Geometry: final body of the model. Coordinates: model frame, mm. Face numbers are marked on the shaded views. A direction names the side the tool comes from. Give positions to 0.01 mm unless a question says otherwise; leave off trailing zeros. Loops run counter-clockwise (first coordinate to the right, second up) from the corner with the lowest first, then second, coordinate; pieces in that order, holes last.
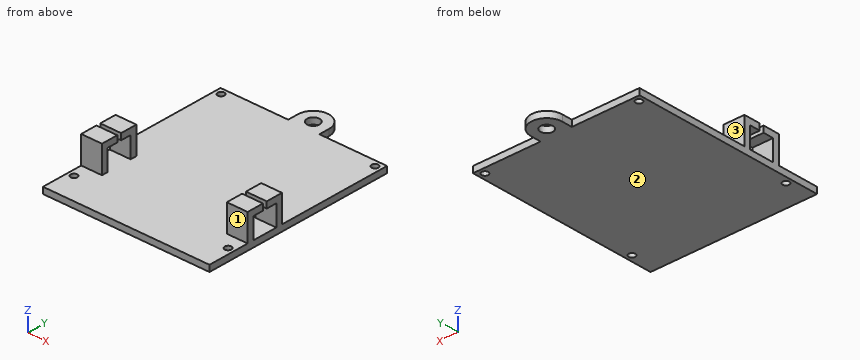
Autodesk Inventor part; units mm, degrees
ref_plane "YZ Plane" through (0, 0, 0) normal (1, 0, 0) x (0, 1, 0)
ref_plane "XZ Plane" through (0, 0, 0) normal (0, 1, 0) x (-1, 0, 0)
ref_plane "XY Plane" through (0, 0, 0) normal (0, 0, 1) x (1, 0, 0)
sketch "Sketch1" plane through (0, 0, 0) normal (0, 0, 1) x (1, 0, 0)
  line L0 (0, 0) -> (80, 0)
  line L1 (80, 0) -> (80, 93)
  line L2 (80, 93) -> (0, 93)
  line L3 (0, 93) -> (0, 0)
  dimension "d0" = 80
  dimension "d1" = 93
extrude "Extrusion1" add sketch "Sketch1" along normal blind 3
sketch "Sketch3" plane through (80, 0, 0) normal (1, 0, 0) x (0, 0, -1)
  line L0 (-3, 0) -> (-3, 93) construction
  line L1 (-3, 20) -> (-16, 20)
  line L2 (-16, 38) -> (-3, 38)
  line L3 (-3, 38) -> (-3, 20) construction
  line L4 (-3, 23) -> (-13, 23)
  line L5 (-13, 35) -> (-3, 35)
  line L6 (0, 0) -> (-3, 0)
  line L7 (-16, 28) -> (-13, 28)
  line L8 (-13, 30) -> (-16, 30)
  line L9 (-16, 20) -> (-16, 28)
  line L10 (-16, 30) -> (-16, 38)
  line L11 (-13, 23) -> (-13, 28)
  line L12 (-13, 30) -> (-13, 35)
  line L13 (-3, 38) -> (-3, 35)
  line L14 (-3, 20) -> (-3, 23)
  point P0 (-13, 19)
  point P1 (-16, 19)
  dimension "d4" = 3
  dimension "d6" = 20
  dimension "d7" = 12
  dimension "d8" = 10
  dimension "d9" = 3
  dimension "d10" = 5
  dimension "d11" = 5
  dimension "d12" = 3
ref_plane "Work Plane1" through (40, 0, 0) normal (1, 0, 0) x (0, 0, -1)
extrude "Extrusion2" add sketch "Sketch3" against normal blind 10
mirror "Mirror1" about plane through (40, 0, 0) normal (1, 0, 0) of "Extrusion2"
sketch "Sketch4" plane through (0, 0, 3) normal (0, 0, 1) x (1, 0, 0)
  circle A0 centre (77, 13) radius 1.6
  line L0 (80, 0) -> (80, 20)
  line L1 (0, 0) -> (80, 0)
  circle A1 centre (77, 90) radius 1.6
  line L2 (80, 93) -> (0, 93)
  dimension "d15" = 3.2
  dimension "d16" = 3
  dimension "d17" = 13
  dimension "d18" = 3
extrude "Extrusion3" cut sketch "Sketch4" against normal through all
mirror "Mirror2" about plane through (40, 0, 0) normal (1, 0, 0) of "Extrusion2", "Extrusion3"
sketch "Sketch5" plane through (0, 0, 0) normal (0, 0, -1) x (-1, 0, 0)
  line L0 (-80, 93) -> (0, 93) construction
  line L1 (-47.5, 93) -> (-32.5, 93)
  line L2 (-32.5, 93) -> (-32.5, 98)
  line L3 (-32.5, 98) -> (-47.5, 98) construction
  line L4 (-47.5, 98) -> (-47.5, 93)
  arc A0 (-32.5, 98) -> (-47.5, 98) centre (-40, 98) ccw
  circle A1 centre (-40, 98) radius 3
  point P0 (0, 0)
  point P1 (-40, 93)
  point P2 (-40, 93)
  dimension "d21" = 6
  dimension "d22" = 15
  dimension "d23" = 5
extrude "Extrusion4" add sketch "Sketch5" against normal blind 3
equation "\"d11\" = d10"
equation "\"d12\" = d4"
equation "\"d18\" = d16"
equation "\"d5\" = d4"
properties part number "Wheel Base"
Item 1: Ray query, probe 1 along Y at (x, z) = (77, 2.35); probe 2 along X at (y, z) = (90, 1.2); probe 3 along Y at (x, z) = (6.5, 4.25). Return the intervals inside material, ascending.
Values follow:
probe 1: y = 0 to 11.4, 14.6 to 88.4, 91.6 to 93
probe 2: x = 0 to 1.4, 4.6 to 75.4, 78.6 to 80
probe 3: y = 20 to 23, 35 to 38
Item 2: Section query D-D on x = 40. Return loops of the section in (y, z).
Values follow:
outline: (0, 0) - (95, 0) - (95, 3) - (0, 3) - close; (101, 0) - (105.5, 0) - (105.5, 3) - (101, 3) - close
Item 3: Set-up query: the marked faces 1, 2 and 3. Return all of +Z, -Z, +X, -X, +Y, -Y with unobstructed straight access to the full face (end or side cutting, diameter ignored); none if empty.
Values follow:
face 1: +Z, +X, -X, -Y
face 2: -Z, +X, -X, +Y, -Y
face 3: +Z, +X, -X, +Y
Item 4: Section query A-A on y = 90. Return loops of the section in (x, z), plus the area to 3 significant figures.
Values follow:
outline: (0, 0) - (1.4, 0) - (1.4, 3) - (0, 3) - close; (4.6, 0) - (75.4, 0) - (75.4, 3) - (4.6, 3) - close; (78.6, 0) - (80, 0) - (80, 3) - (78.6, 3) - close
area: 221 mm2
Item 5: Section query C-C on x = 77. Return loops of the section in (y, z).
Values follow:
outline: (0, 0) - (11.4, 0) - (11.4, 3) - (0, 3) - close; (14.6, 0) - (88.4, 0) - (88.4, 3) - (38, 3) - (38, 16) - (30, 16) - (30, 13) - (35, 13) - (35, 3) - (23, 3) - (23, 13) - (28, 13) - (28, 16) - (20, 16) - (20, 3) - (14.6, 3) - close; (91.6, 0) - (93, 0) - (93, 3) - (91.6, 3) - close
Item 6: Section query B-B on z = 11.75. Return loops of the section in (x, y), plus the area to 3 significant figures.
Values follow:
outline: (0, 20) - (10, 20) - (10, 23) - (0, 23) - close; (0, 35) - (10, 35) - (10, 38) - (0, 38) - close; (70, 20) - (80, 20) - (80, 23) - (70, 23) - close; (70, 35) - (80, 35) - (80, 38) - (70, 38) - close
area: 120 mm2
Item 7: Pin query (flat end, axial travel): pin 1 (0.9 mm diameter, centred on x = 21, z = 1.5, fed in from +Y); pin 2 (5 mm diameter, centred on x = 3, z = 6.5, fed in from -Y); pin 3 (9.5 mm diameter, centred on x = 40, y = 98, fed in from +Z). Return the tip coordinate at first contact, or that it passes through.
Values follow:
pin 1: stops at y = 93
pin 2: stops at y = 20
pin 3: stops at z = 3
